Could you check a few things on this model? Use its own coordinates, in mm. A direction names the side the tool comes from. Coordinates: 2 decimals unless noted, no trailing zeros. Write each loop counter-clockwise with the first axis right and the second up, starting at its lowest first coordinate (ties: lowest second). Pieces come first, ordered by that corner, then holes. Notation, with made-up numbers: M 32.5,83 L 89.5,83 A31 cw 89.5,118 Z; hole C 65,30.5 d2. An arc over 180 degrees is marked long. Answer as CSV lines item,"result". Start each with the question number.
Item 1: On a 3-axis mill with a long thin cutter (end or side, diameter ignored), from which of +Z, -Z, +X, -X, +Y, -Y can I reach the whole of each face in a straight line? I mean faces 1 (the flat face through (1, 6, -2)), 2 (the flat face through (69, 8, -2)), 3 (the flat face through (-69, 8, -2)), 4 (the flat face through (68.5, 53, -73)). Say none if no direction works.
Item 2: Suppose I cut it at A-A, the plane x = 56. Write out the boundary of the cut face in (y, z), and give its area (3 significant figures).
Item 3: Suppose I cut it at B-B, the plane z = -96. Write out the boundary of the cut face in (x, y), and give its area (3 significant figures).
Item 4: We'd pull the mould along Y, two halves only. Please class faces 5 (the flat face through (1, 17, -2)), 6 (the flat face through (1, 10, -2)), 7 (the flat face through (1, 8, -4)), 8 (the flat face through (72, 50.5, -73)): +Y half, -Y half, draft (parallel to the pull), parting line (faces both ways), or undercut.
Item 5: I'm going to push flat-ended pins straight in: P1, Ø10, axis at x = 37.5, z = -66.5, coming from the -Y side; P2, Ø1.5, axis at y = 44, z = -15.5, coming from the -X side (3 decimals); P3, Ø3, axis at x = -32, y = 14, coming from the -Z side; P4, Ø3, axis at y = 7, z = -2.5, coming from the -X side. Where does each tip first touch, or does it pass through?
Item 6: Suppose I cut it at C-C, the plane y = 39. Write out the boundary of the cut face in (x, z), and give its area (3 significant figures).
Item 7: If I drill on line 1 along Y through (x, z) = (-73, 2.75); line 2 along Y through (x, z) = (3.5, -142); line 3 along X through (y, z) = (51, -17.5), over which ranges is the centre line in solid material (lowest first)? Write a range as [from, to].
```python
from build123d import *

# Parameters (mm, degrees)
SKETCH1_W           = 160
SKETCH1_H           = 55
BOSS_EXTRUDE1_DEPTH = 5
SKETCH4_W           = 138
SKETCH4_H           = 4
BOSS_EXTRUDE3_DEPTH = 4
FILLET1_R           = 2
CUT_EXTRUDE1_REACH  = 99.211
SKETCH10_R          = 1.25
BOSS_EXTRUDE4_DEPTH = 149


with BuildPart() as part:
    # Sketch1 → Boss-Extrude1 (new body)
    with BuildSketch(Plane.XY):
        with Locations((0, 27.5)):
            Rectangle(SKETCH1_W, SKETCH1_H)
    extrude(amount=BOSS_EXTRUDE1_DEPTH)

    # Sketch4 → Boss-Extrude3 (add)
    with BuildSketch(Plane(origin=(0, 0, 0), x_dir=(-1, 0, 0), z_dir=(0, 0, -1))):
        with Locations((0, 15)):
            Rectangle(SKETCH4_W, SKETCH4_H)
        with Locations((0, 8)):
            Rectangle(SKETCH4_W, SKETCH4_H)
    extrude(amount=BOSS_EXTRUDE3_DEPTH)

    # Fillet1
    fillet1_edges = [part.edges().sort_by_distance(p)[0] for p in [
        (-80, 27.5, 5),
        (0, 0, 5),
        (80, 27.5, 5),
        (0, 55, 5),
        (80, 0, 2.5),
        (-80, 0, 2.5),
        (-80, 55, 2.5),
        (80, 55, 2.5),
    ]]
    fillet(fillet1_edges, radius=FILLET1_R)

    # Sketch10 → Cut-Extrude1 (cut, up to next)
    with BuildSketch(Plane(origin=(0, 0, 0), x_dir=(-1, 0, 0), z_dir=(0, 0, -1)), mode=Mode.PRIVATE) as cut_extrude1_sk1:
        with Locations((-73, 31)):
            Circle(SKETCH10_R)
    cut_extrude1_tool1 = extrude(cut_extrude1_sk1.sketch, amount=-CUT_EXTRUDE1_REACH, mode=Mode.PRIVATE) & part.part
    cut_extrude1 = cut_extrude1_tool1.solids().sort_by_distance((73, 31, 0))[0]
    add(cut_extrude1, mode=Mode.SUBTRACT)

    # Mirror1: Cut-Extrude1 across plane
    add(cut_extrude1.mirror(Plane(origin=(0, 0, 0), x_dir=(0, 0, 1), z_dir=(1, 0, 0))), mode=Mode.SUBTRACT)

    # Sketch13 → Boss-Extrude4 (add)
    with BuildSketch(Plane(origin=(0, 0, 0), x_dir=(-1, 0, 0), z_dir=(0, 0, -1))):
        Polygon((-68.5, 55), (-68.5, 50.5), (-76.5, 50.5), (-76.5, 48.5), (-68.5, 48.5), (-68.5, 45), (68.5, 45), (68.5, 48.5), (76.5, 48.5), (76.5, 50.5), (68.5, 50.5), (68.5, 55), align=None)
    extrude(amount=BOSS_EXTRUDE4_DEPTH)


solid = part.part
```
Ans:
1,face 1,"-Z, +X, -X, -Y"
1,face 2,"-Z, +X, -Y"
1,face 3,"-Z, -X, -Y"
1,face 4,"-Z, +X, +Y"
2,outline,"M 0,0 L 6,0 L 6,-4 L 10,-4 L 10,0 L 13,0 L 13,-4 L 17,-4 L 17,0 L 45,0 L 45,-149 L 55,-149 L 55,3 A2 ccw 53,5 L 2,5 A2 ccw 0,3 Z"
2,area,"1,800 mm^2"
3,outline,"M -76.5,48.5 L -68.5,48.5 L -68.5,45 L 68.5,45 L 68.5,48.5 L 76.5,48.5 L 76.5,50.5 L 68.5,50.5 L 68.5,55 L -68.5,55 L -68.5,50.5 L -76.5,50.5 Z"
3,area,"1,400 mm^2"
4,face 5,"undercut"
4,face 6,"undercut"
4,face 7,"draft"
4,face 8,"+Y half"
5,P1,"stops at y = 45"
5,P2,"passes through"
5,P3,"stops at z = -4"
5,P4,"stops at x = -69"
6,outline,"M -80,0 L 80,0 L 80,3 A2 ccw 78,5 L -78,5 A2 ccw -80,3 Z"
6,area,"798 mm^2"
7,line 1,"y = [0, 29.75], [32.25, 55]"
7,line 2,"y = [45, 55]"
7,line 3,"x = [-68.5, 68.5]"
